The model under review builds one solid part; all positions refer to its coordinate system, in mm. A direction names the side the tool comes from. Round coordinates to 2 decimals unless told otherwise and drop trailing zeros. Order: outer loops, then holes, each group sorted by start corner. A loop starts at its lowest first (then second) coordinate and runs counter-clockwise, first axis right, second up. Notation, with made-up numbers: M 74,32.5 L 118,32.5 A21 cw 118,51.5 Z; hole C 71.5,20 d8. An arc over 180 degrees is marked long. One line per item, written item: value. Start each with the question number.
from build123d import *

# Parameters (mm, degrees)
F1_DEPTH = 470
F3_DEPTH = 8
F5_DEPTH = 8


with BuildPart() as f1:
    # F0 (on Top) → F1 (new body)
    with BuildSketch(Plane.XY):
        Polygon((0, 50), (0, 0), (50, 0), (50, 8), (8, 8), (8, 50), align=None)
    extrude(amount=F1_DEPTH)

    # F2 (on face) → F3 (cut, through all)
    with BuildSketch(Plane.XZ):
        Polygon((50, 470), (0, 470), (50, 420), align=None)
    extrude(amount=-F3_DEPTH, mode=Mode.SUBTRACT)

    # F4 (on face) → F5 (cut, through all)
    with BuildSketch(Plane(origin=(0, 0, 0), x_dir=(0, -1, 0), z_dir=(-1, 0, 0))):
        Polygon((-50, 420), (0, 470), (-8, 470), (-50, 470), align=None)
    extrude(amount=-F5_DEPTH, mode=Mode.SUBTRACT)


solid = f1.part
Item 1: Clearance check with flat-ended pins moving along their axes: P1, Ø4, axis at x = 34, z = 260, coming from the +Y side; P2, Ø21, axis at y = 37, z = 294.5, coming from the +X side; P3, Ø8, axis at x = 38, z = 270.5, coming from the -Y side; P4, Ø3, axis at x = 5.5, y = 6, coming from the +Z side. State where each tip first meets the part, or that it passes through.
Item 2: Consider section C-C, the plane x = 26. Give the boundary of the cut face in (y, z).
Item 3: Machinability: for faces 1 (the flat face through (0, 25, 232)), 2 (the flat face through (29, 8, 228)), which of the approach directions +Z, -Z, +X, -X, +Y, -Y give a long, thin tool a straight path to every point of the face, cutting with its end or side? Answer none if there is none.
Item 4: Consider section B-B, the plane y = 13.5. Give the boundary of the cut face in (x, z), then the cut area to 3 significant figures.
Item 5: Wall thickness on L1, parallel to Y at x = 8.5, z = 212.5; L2, parallel to Z at x = 40.5, y = 4.5: over which ranges is each line inside the solid? List them lowest first.
Item 6: Consider section D-D, the plane z = 441. Give the boundary of the cut face in (x, y), then the cut area to 3 significant figures.
Item 7: Consider section A-A, the plane z = 148.5. Give the boundary of the cut face in (x, y), then the cut area to 3 significant figures.
Computed:
1. P1: stops at y = 8
1. P2: stops at x = 8
1. P3: stops at y = 0
1. P4: stops at z = 465.28
2. outline: M 0,0 L 8,0 L 8,444 L 0,444 Z
3. face 1: +Z, -Z, -X, +Y, -Y
3. face 2: +Z, -Z, +X, +Y
4. outline: M 0,0 L 8,0 L 8,456.5 L 0,456.5 Z
4. area: 3,650 mm^2
5. L1: y = 0 to 8
5. L2: z = 0 to 429.5
6. outline: M 0,0 L 29,0 L 29,8 L 8,8 L 8,29 L 0,29 Z
6. area: 400 mm^2
7. outline: M 0,0 L 50,0 L 50,8 L 8,8 L 8,50 L 0,50 Z
7. area: 736 mm^2
